Could you check a few things on this model? Use its own coordinates, in mm. Give positions to 0.01 mm unless a question says otherwise; leave off trailing zeros.
from build123d import *

# Parameters (mm, degrees)
F0_R     = 7.75
F1_DEPTH = 10
F4_R     = 2.75
F5_DEPTH = 10


with BuildPart() as f1:
    # F0 (on Top) → F1 (new body)
    with BuildSketch(Plane.XY):
        Circle(F0_R)
    extrude(amount=F1_DEPTH)

    # F2 (on Front) → F3 (revolve)
    with BuildSketch(Plane.XZ):
        with BuildLine():
            ThreePointArc((0, 8.283929), (18.358036, 26.641964), (0, 45))
            Line((0, 45), (0, 8.283929))
        make_face()
    revolve(axis=Axis((0, 0, 26.641964), (0, 0, -1)))

    # F4 (on face) → F5 (cut)
    with BuildSketch(Plane(origin=(0, 0, 0), x_dir=(1, 0, 0), z_dir=(0, 0, -1))):
        Circle(F4_R)
    extrude(amount=-F5_DEPTH, mode=Mode.SUBTRACT)

    # F6 (on Front) → F7 (revolve, cut)
    with BuildSketch(Plane.XZ):
        with BuildLine():
            ThreePointArc((2.75, 10), (0, 12.75), (-2.75, 10))
            Line((-2.75, 10), (2.75, 10))
        make_face()
    revolve(axis=Axis((0, 0, 10), (1, 0, 0)), mode=Mode.SUBTRACT)


solid = f1.part
Item 1: We'd pull the mould along Y, two halves only. Please class faces 1 (the flat face through (0, -3, 0)), 2 (the cylindrical face through (-1.009, 7.684, 4.93)), 3 (the cylindrical face through (-0.596, 2.685, 4.93)): +Y half, -Y half, draft (parallel to the pull), parting line (faces both ways), or undercut.
Findings:
face 1: draft
face 2: parting line
face 3: undercut
Item 2: For pin 1 (4 mm diameter, centred on x = 14.5, z = 16.5, fed in from -Y); pin 2 (3.5 mm diameter, centred on x = 0, y = 0, fed in from -Z); pin 3 (1.5 mm diameter, centred on y = 9, z = 21, fed in from -X); pin 4 (6 mm diameter, centred on y = 12, z = 7, fed in from -X), each with a flat end and sliding along its axis, tell me the tip position at first contact or that it passes through.
Findings:
pin 1: stops at y = -9.52
pin 2: stops at z = 12.12
pin 3: stops at x = -15.48
pin 4: passes through
Item 3: Please list where these lines run through material, in increasing order: line 1 along Y through (x, z) = (0, 3.75); line 2 along Y through (x, z) = (-7, 29); line 3 along X through (y, z) = (12, 30).
Findings:
line 1: y = -7.75 to -2.75, 2.75 to 7.75
line 2: y = -16.81 to 16.81
line 3: x = -13.48 to 13.48
